Autodesk Inventor part; units mm, degrees
ref_plane "YZ Plane" through (0, 0, 0) normal (1, 0, 0) x (0, 1, 0)
ref_plane "XZ Plane" through (0, 0, 0) normal (0, 1, 0) x (-1, 0, 0)
ref_plane "XY Plane" through (0, 0, 0) normal (0, 0, 1) x (1, 0, 0)
sketch "Sketch1" plane through (0, 0, 0) normal (0, 1, 0) x (-1, 0, 0)
  circle A0 centre (110.109, -133.985) radius 57.15
  circle A1 centre (110.109, -133.985) radius 50.8
  circle A2 centre (110.109, -133.985) radius 69.85
  line L0 (206.4385, -159.385) -> (175.1771, -159.385)
  line L1 (206.4385, -159.385) -> (206.4385, -108.585)
  line L2 (206.4385, -108.585) -> (175.1771, -108.585)
  point P0 (0, 0)
  dimension "d51" = 139.7
  dimension "d11" = 114.3
  dimension "d12" = 101.6
extrude "Extrusion11" add sketch "Sketch1" against normal blind 25.4 contours A0 | A1 | A2 | A2 L2 L1 L0
extrude "Extrusion12" add sketch "Sketch1" along normal blind 12.7 contours A0 | A1
chamfer "Chamfer1" distance 3.175 angle 45 1 edges at (-52.959, 12.7, -133.985)
chamfer "Chamfer2" distance 6.35 angle 45 1 edges at (-40.259, -25.4, -133.985)
fillet "Fillet2" radius 12.7 2 edges at (-206.4385, -25.4, -133.985) (-206.4385, 0, -133.985)
sketch "Sketch5" plane through (-175.1771, -19.05, -108.585) normal (0, 0, 1) x (1, 0, 0)
  arc A0 (-18.5614, 19.05) -> (-18.5614, -6.35) centre (-18.5614, 6.35) ccw
  circle A1 centre (-18.5614, 6.35) radius 6.35
  point P0 (175.1771, 19.05)
  dimension "d63" = 12.7
extrude "Extrusion13" add sketch "Sketch5" along normal blind 12.7
sketch "Sketch6" plane through (-175.1771, -19.05, -159.385) normal (0, 0, -1) x (-1, 0, 0)
  arc A0 (18.5614, -6.35) -> (18.5614, 19.05) centre (18.5614, 6.35) ccw
  circle A1 centre (18.5614, 6.35) radius 6.35
  point P0 (-175.1771, 19.05)
  dimension "d66" = 12.7
extrude "Extrusion14" add sketch "Sketch6" along normal blind 12.7
properties part number "Access Hatch"
Part model, mm, in its own coordinate system. A direction names the side the tool comes from. Give positions to 0.01 mm unless a question says otherwise; leave off trailing zeros. Order: outer loops, then holes, each group sorted by start corner. A loop starts at its lowest first (then second) coordinate and runs counter-clockwise, first axis right, second up. Notation, with made-up numbers: M 8,-35 L 33,-35 A31 cw 33,-1 Z; hole C 7,21 d4. An arc over 180 degrees is marked long. Use a Markdown table: item, result. Add a question column.
(1) 3-axis set-ups, long thin cutter, end or side, ignore diameter. For faces 1 (the face through (-194, -13, -172.085)), 2 (the face through (-194, -13, -95.885)), 3 (the face through (-187.6, -15.3, -159.385)): which of +Z, -Z, +X, -X, +Y, -Y reach the whole face in a straight line?
(2) Saw through at A-A, the plane x = -178. Give the cut face in (y, z) (3 decimals), and give its area (3 significant figures).
(3) Mould opens along X. For faces 4 (the face through (-190.32, -18.05, -102.32)), 5 (the face through (-119, -25.4, -133)), 6 (the face through (-135.107, 12.501, -85.924)) say: +X half, -X half, draft (parallel to the pull), parting line (faces both ways), or undercut.
(4) Probe line 1 along X through (y, z) = (-11, -170.5); line 2 along Z through (x, y) = (-110, -14); line 3 along X through (y, z) = (-12, -102.5). List the from-to ranges inside material, lowest first. Write a range as [from, to].
(5) Drop flat-ended pins along their axis: P1, Ø10, axis at y = -1.5, z = -112.5, coming from the -X side; P2, Ø8, axis at x = -167.5, y = -8.5, coming from the -Z side; P3, Ø2, axis at x = -72.5, y = -19, coming from the +Z side. Give the stop position or say it passes through.
Answer key:
| question | item | result |
|---|---|---|
| 1 | face 1 | -Z, -X, +Y, -Y |
| 1 | face 2 | +Z, -X, +Y, -Y |
| 1 | face 3 | -Z |
| 2 | outline | M -25.4,-159.385 L 0,-159.385 L 0,-108.585 L -25.4,-108.585 Z |
| 2 | area | 1,290 mm^2 |
| 3 | face 4 | undercut |
| 3 | face 5 | draft |
| 3 | face 6 | parting line |
| 4 | line 1 | [-199.86, -187.62], [-169.65, -50.56] |
| 4 | line 2 | [-203.83, -64.14] |
| 4 | line 3 | [-200.05, -187.43], [-172.46, -47.76] |
| 5 | P1 | x = -204.82 |
| 5 | P2 | z = -179.02 |
| 5 | P3 | z = -74.5 |
